For this review, take the finished solid that the model builds, in its own axes (mm). A direction names the side the tool comes from. Give positions to 0.01 mm unless a question says otherwise; leave off trailing zeros. Write each loop counter-clockwise with the first axis right and the second up, starting at its lowest first coordinate (ties: lowest second). Pieces come first, ordered by that corner, then holes.
Q1. We need section C-C (y = -50.8). Write out the cut boundary in (x, z) (3 decimals).
Q2. We need section D-D (z = 2.25). Give the number of separate pieces and of enclosed holes in the cut face, then the cut area to 3 significant figures.
Q3. We need section A-A (x = 50.8). Write out the cut boundary in (y, z) (3 decimals), then the cut area to 3 significant figures.
Q4. Mouldability with a two-part tool opening along Y and no side actions: class faces 1 (the flat face through (-1, 76.2, 6)), 2 (the cylindrical face through (-53.14, -48.654, 5.916)), 3 (the flat face through (-1, 73, 12)), 4 (the flat face through (0.1, 28.8, 5.08)) as released by +Y, released by -Y, zero draft, split by the parting line, or undercut.
Q5. We need section B-B (y = 31.4). Write out the cut boundary in (x, z) (3 decimals).
Q6. For line 1 (Y direction, x = 19.5, z = 9.75); line 2 (Y direction, x = 0, z = 7); line 3 (X direction, y = -65, z = 8), list the stretches that pass through material, from the lowest coordinate up.
Q7. Machinability: for faces 5 (the flat face through (-1, -47, 12)), 6 (the cylindrical face through (-30.89, 27.526, 2.504)), 7 (the flat face through (-1, -34, 8.825)), which of the approach directions +Z, -Z, +X, -X, +Y, -Y give a long, thin tool a straight path to every point of the face, cutting with its end or side? Answer none if there is none.
Q8. Insertion check: P1, Ø9.5, axis at x = -14, y = 65, coming from the +Z side; P2, Ø2.5, axis at x = 33.5, y = -29.5, coming from the -Z side; P3, Ø3, axis at x = -51, y = -32.5, coming from the +Z side (3 decimals). Each pin has a flat end and moves straight along its axis. Give the tip position at first contact, or say it passes through.
```python
from build123d import *

# Parameters (mm, degrees)
SKETCH1_W           = 152.4
SKETCH1_H           = 152.4
SKETCH1_R           = 3.175
BOSS_EXTRUDE1_DEPTH = 12
SKETCH2_W           = 152.4
SKETCH2_H           = 12
SKETCH2_R           = 2.38125
CUT_EXTRUDE1_DEPTH  = 3.175
SKETCH3_R           = 2.38125
CUT_EXTRUDE2_DEPTH  = 109.429147373
SKETCH5_R           = 3.96875
CUT_EXTRUDE7_DEPTH  = 5.08


with BuildPart() as part:
    # Sketch1 → Boss-Extrude1 (new body)
    with BuildSketch(Plane.XY):
        Rectangle(SKETCH1_W, SKETCH1_H)
        with Locations((-50.8, 50.8)):
            Circle(SKETCH1_R, mode=Mode.SUBTRACT)
        with Locations((-50.8, -50.8)):
            Circle(SKETCH1_R, mode=Mode.SUBTRACT)
        with Locations((50.8, 50.8)):
            Circle(SKETCH1_R, mode=Mode.SUBTRACT)
        with Locations((50.8, -50.8)):
            Circle(SKETCH1_R, mode=Mode.SUBTRACT)
    extrude(amount=BOSS_EXTRUDE1_DEPTH)

    # Sketch2 → Cut-Extrude1 (cut)
    # profile 1 of 4: a face of its own
    with BuildSketch(Plane.XY.offset(12)):
        with Locations((0, -31.4)):
            Rectangle(SKETCH2_W, SKETCH2_H)
        with Locations((0, -31.4)):
            Circle(SKETCH2_R, mode=Mode.SUBTRACT)
        with Locations((-31.75, -31.4)):
            Circle(SKETCH2_R, mode=Mode.SUBTRACT)
        with Locations((31.75, -31.4)):
            Circle(SKETCH2_R, mode=Mode.SUBTRACT)
    # profile 2 of 4: a face of its own
    with BuildSketch(Plane.XY.offset(12)):
        with Locations((0, 31.4)):
            Rectangle(SKETCH2_W, SKETCH2_H)
        with Locations((0, 31.4)):
            Circle(SKETCH2_R, mode=Mode.SUBTRACT)
        with Locations((31.75, 31.4)):
            Circle(SKETCH2_R, mode=Mode.SUBTRACT)
        with Locations((-31.75, 31.4)):
            Circle(SKETCH2_R, mode=Mode.SUBTRACT)
    # profile 3 of 4: a face of its own
    with BuildSketch(Plane.XY.offset(12)):
        with Locations((0, 63.5)):
            Rectangle(SKETCH2_W, SKETCH2_H)
        with Locations((-31.75, 63.5)):
            Circle(SKETCH2_R, mode=Mode.SUBTRACT)
        with Locations((0, 63.5)):
            Circle(SKETCH2_R, mode=Mode.SUBTRACT)
        with Locations((31.75, 63.5)):
            Circle(SKETCH2_R, mode=Mode.SUBTRACT)
    # profile 4 of 4: a face of its own
    with BuildSketch(Plane.XY.offset(12)):
        with Locations((0, -63.5)):
            Rectangle(SKETCH2_W, SKETCH2_H)
        with Locations((0, -63.5)):
            Circle(SKETCH2_R, mode=Mode.SUBTRACT)
        with Locations((-31.75, -63.5)):
            Circle(SKETCH2_R, mode=Mode.SUBTRACT)
        with Locations((31.75, -63.5)):
            Circle(SKETCH2_R, mode=Mode.SUBTRACT)
    extrude(amount=-CUT_EXTRUDE1_DEPTH, mode=Mode.SUBTRACT)

    # Sketch3 → Cut-Extrude2 (cut, through all)
    with BuildSketch(Plane.XY.offset(12)):
        with Locations((-31.75, 63.5)):
            Circle(SKETCH3_R)
        with Locations((0, 63.5)):
            Circle(SKETCH3_R)
        with Locations((31.75, 63.5)):
            Circle(SKETCH3_R)
        with Locations((-31.75, 31.4)):
            Circle(SKETCH3_R)
        with Locations((0, 31.4)):
            Circle(SKETCH3_R)
        with Locations((31.75, 31.4)):
            Circle(SKETCH3_R)
        with Locations((-31.75, -31.4)):
            Circle(SKETCH3_R)
        with Locations((0, -31.4)):
            Circle(SKETCH3_R)
        with Locations((31.75, -31.4)):
            Circle(SKETCH3_R)
        with Locations((-31.75, -63.5)):
            Circle(SKETCH3_R)
        with Locations((0, -63.5)):
            Circle(SKETCH3_R)
        with Locations((31.75, -63.5)):
            Circle(SKETCH3_R)
    extrude(amount=-CUT_EXTRUDE2_DEPTH, mode=Mode.SUBTRACT)

    # Sketch5 → Cut-Extrude7 (cut)
    with BuildSketch(Plane(origin=(0, 0, 0), x_dir=(-1, 0, 0), z_dir=(0, 0, -1))):
        with Locations((31.75, -63.5)):
            Circle(SKETCH5_R)
        with Locations((0, -63.5)):
            Circle(SKETCH5_R)
        with Locations((-31.75, -63.5)):
            Circle(SKETCH5_R)
        with Locations((-31.75, -31.4)):
            Circle(SKETCH5_R)
        with Locations((0, -31.4)):
            Circle(SKETCH5_R)
        with Locations((31.75, -31.4)):
            Circle(SKETCH5_R)
        with Locations((31.75, 31.4)):
            Circle(SKETCH5_R)
        with Locations((0, 31.4)):
            Circle(SKETCH5_R)
        with Locations((-31.75, 31.4)):
            Circle(SKETCH5_R)
        with Locations((-31.75, 63.5)):
            Circle(SKETCH5_R)
        with Locations((0, 63.5)):
            Circle(SKETCH5_R)
        with Locations((31.75, 63.5)):
            Circle(SKETCH5_R)
    extrude(amount=-CUT_EXTRUDE7_DEPTH, mode=Mode.SUBTRACT)


solid = part.part
```
Computed:
1. outline: (-76.2, 0) - (-53.975, 0) - (-53.975, 12) - (-76.2, 12) - close; (-47.625, 0) - (47.625, 0) - (47.625, 12) - (-47.625, 12) - close; (53.975, 0) - (76.2, 0) - (76.2, 12) - (53.975, 12) - close
2. separate pieces: 1
2. enclosed holes: 16
2. area: 22,500 mm2
3. outline: (-76.2, 0) - (-53.975, 0) - (-53.975, 12) - (-57.5, 12) - (-57.5, 8.825) - (-69.5, 8.825) - (-69.5, 12) - (-76.2, 12) - close; (-47.625, 0) - (47.625, 0) - (47.625, 12) - (37.4, 12) - (37.4, 8.825) - (25.4, 8.825) - (25.4, 12) - (-25.4, 12) - (-25.4, 8.825) - (-37.4, 8.825) - (-37.4, 12) - (-47.625, 12) - close; (53.975, 0) - (76.2, 0) - (76.2, 12) - (69.5, 12) - (69.5, 8.825) - (57.5, 8.825) - (57.5, 12) - (53.975, 12) - close
3. area: 1,520 mm2
4. face 1: released by +Y
4. face 2: undercut
4. face 3: zero draft
4. face 4: undercut
5. outline: (-76.2, 0) - (-35.719, 0) - (-35.719, 5.08) - (-34.131, 5.08) - (-34.131, 8.825) - (-76.2, 8.825) - close; (-29.369, 5.08) - (-27.781, 5.08) - (-27.781, 0) - (-3.969, 0) - (-3.969, 5.08) - (-2.381, 5.08) - (-2.381, 8.825) - (-29.369, 8.825) - close; (2.381, 5.08) - (3.969, 5.08) - (3.969, 0) - (27.781, 0) - (27.781, 5.08) - (29.369, 5.08) - (29.369, 8.825) - (2.381, 8.825) - close; (34.131, 5.08) - (35.719, 5.08) - (35.719, 0) - (76.2, 0) - (76.2, 8.825) - (34.131, 8.825) - close
6. line 1: y = -76.2 to -69.5, -57.5 to -37.4, -25.4 to 25.4, 37.4 to 57.5, 69.5 to 76.2
6. line 2: y = -76.2 to -65.88, -61.12 to -33.78, -29.02 to 29.02, 33.78 to 61.12, 65.88 to 76.2
6. line 3: x = -76.2 to -33.6, -29.9 to -1.85, 1.85 to 29.9, 33.6 to 76.2
7. face 5: +Z, +X, -X, +Y, -Y
7. face 6: -Z
7. face 7: +Z, +X, -X
8. P1: stops at z = 12
8. P2: stops at z = 5.08
8. P3: stops at z = 8.825
